from build123d import *

# Parameters (mm, degrees)
PAD_DEPTH         = 90
FILLET_R          = 6
CYLINDER_R        = 12
CYLINDER_DEPTH    = 90
CYLINDER001_R     = 12
CYLINDER001_DEPTH = 90


with BuildPart() as part:
    # Sketch → Pad (new body)
    with BuildSketch(Plane.XY):
        Polygon((-136.659612, 0), (113.340388, 0), (113.340388, 12), (63.340388, 12), (63.340388, 66.999997), (51.340388, 66.999997), (51.340388, 15), (24.340388, 13.5), (24.340388, 12), (9.340388, 12), (6.340388, 30), (6.340388, 67), (-5.659612, 67), (-5.659612, 12), (-136.659612, 12), align=None)
    extrude(amount=PAD_DEPTH)

    # Fillet
    fillet_edges = [part.edges().sort_by_distance(p)[0] for p in [
        (-136.659612, 12, 45),
        (-71.159612, 12, 90),
        (-71.159612, 12, 0),
        (-5.659612, 67, 45),
        (-5.659612, 39.5, 0),
        (-5.659612, 39.5, 90),
        (-136.659612, 6, 0),
        (-136.659612, 6, 90),
    ]]
    fillet(fillet_edges, radius=FILLET_R)

    # Cylinder → Cylinder (join)
    with BuildSketch(Plane(origin=(-5.659612, 12, 90), x_dir=(-1, 0, 0), z_dir=(0, 0, -1))):
        Circle(CYLINDER_R)
    extrude(amount=CYLINDER_DEPTH)

    # Cylinder001 → Cylinder001 (join)
    with BuildSketch(Plane(origin=(63.340388, 12, 90), x_dir=(-1, 0, 0), z_dir=(0, 0, -1))):
        Circle(CYLINDER001_R)
    extrude(amount=CYLINDER001_DEPTH)


solid = part.part
Here's how the part is built. I have some questions about the finished solid (model axes, mm). A direction names the side the tool comes from. Round coordinates to 2 decimals unless told otherwise and drop trailing zeros. Write each loop counter-clockwise with the first axis right and the second up, starting at its lowest first coordinate (ties: lowest second). Pieces come first, ordered by that corner, then holes.
1. I need wall thicknesses on L1, parallel to X at y = 33, z = 84; L2, parallel to Y at x = -65, z = 19.5; L3, parallel to X at y = 18, z = 70. Which ranges of each line are inside material? Lowest first, please.
2. Suppose I cut it at B-B (z = 40.5). List the corners of the cut face in (x, y) for me.
3. Suppose I cut it at A-A (y = 56). List the corners of the cut face in (x, z) for me, and give its area (3 significant figures).
4. For faces 1 (the flat face through (51.34, 41, 44)), 2 (the flat face through (-73, 12, 44)), 3 (the flat face through (95, 12, 44)), which set-ups out of +Z, -Z, +X, -X, +Y, -Y let a thin tool reach every point of the face, with its end or its side?
5. Will these pins go through, and if not, where does the flat tip stop? pin 1 Ø1.5 at (x, z) = (-19.5, 10.5) entering from -Y; pin 2 Ø7.5 at (x, z) = (16.5, 42) entering from +Y; pin 3 Ø5 at (y, z) = (46, 15.5) entering from +X; pin 4 Ø5 at (x, z) = (38.5, 67.5) entering from +Y.
6. Suppose I cut it at C-C (x = 91.5). List the corners of the cut face in (y, z) for me, and give its area (3 significant figures).
7. If we mould it in two halves opening along X, with no side actions, what happens to faces 4 (the flat face through (7.861, 20.874, 44.37)), 5 (the flat face through (19, 11, 0)), 6 (the flat face through (63.34, 45, 44))? For each: released by +X, released by -X, zero draft, split by the parting line, or undercut.
8. Suppose I cut it at D-D (x = -44). List the corners of the cut face in (y, z) for me.
Answer sheet:
1. L1: x = -5.66 to 6.34, 51.34 to 63.34
1. L2: y = 0 to 12
1. L3: x = -16.05 to 8.34, 51.34 to 73.73
2. outline: (-136.66, 0) - (113.34, 0) - (113.34, 12) - (75.34, 12) arc R12 ccw to (63.34, 24) - (63.34, 67) - (51.34, 67) - (51.34, 15) - (24.34, 13.5) - (24.34, 12) - (9.34, 12) - (6.34, 30) - (6.34, 67) - (0.34, 67) arc R6 ccw to (-5.66, 61) - (-5.66, 24) arc R12 ccw to (-17.66, 12) - (-130.66, 12) arc R6 ccw to (-136.66, 6) - close
3. outline: (-5.66, 6) arc R6 ccw to (0.34, 0) - (6.34, 0) - (6.34, 90) - (0.34, 90) arc R6 ccw to (-5.66, 84) - close; (51.34, 0) - (63.34, 0) - (63.34, 90) - (51.34, 90) - close
3. area: 2,140 mm2
4. face 1: +Z, -Z, +Y
4. face 2: +Z, -Z, -X, +Y
4. face 3: +Z, -Z, +X, +Y
5. pin 1: stops at y = 0
5. pin 2: stops at y = 12
5. pin 3: stops at x = 63.34
5. pin 4: stops at y = 14.43
6. outline: (0, 0) - (12, 0) - (12, 90) - (0, 90) - close
6. area: 1,080 mm2
7. face 4: undercut
7. face 5: zero draft
7. face 6: released by +X
8. outline: (0, 0) - (6, 0) arc R6 ccw to (12, 6) - (12, 84) arc R6 ccw to (6, 90) - (0, 90) - close
